Geometry check sheet. Reference: the model listing, model coordinates, mm. A direction names the side the tool comes from. Give positions to 0.01 mm unless a question says otherwise; leave off trailing zeros. Order: outer loops, then holes, each group sorted by start corner. A loop starts at its lowest first (then second) coordinate and runs counter-clockwise, first axis right, second up. Notation, with made-up numbers: M 84.25,88 L 99.25,88 A22 ccw 99.25,99 Z; hole C -25,66.25 d8. An arc over 180 degrees is marked long. One line per question, with ' | ' between items. Start each with the question number.
from build123d import *

# Parameters (mm, degrees)
SKETCH052_W     = 14
SKETCH052_H     = 6
PAD022_DEPTH    = 2
PAD023_DEPTH    = 1.8
PAD024_DEPTH    = 2
SKETCH056_W     = 3
SKETCH056_H     = 3
POCKET025_DEPTH = 2


with BuildPart() as part:
    # Sketch052 → Pad022 (new body)
    with BuildSketch(Plane(origin=(232, -0.5, 0.8), x_dir=(0, 1, 0), z_dir=(1, 0, 0))):
        with Locations((-52.22, 6.7)):
            Rectangle(SKETCH052_W, SKETCH052_H)
    extrude(amount=PAD022_DEPTH)

    # Sketch053 (on Face6 of Pad022) → Pad023 (join)
    with BuildSketch(Plane.YZ.offset(234)):
        with BuildLine():
            ThreePointArc((-54.97, 9.25), (-56.72, 7.5), (-54.97, 5.75))
            Line((-54.97, 5.75), (-50.47, 5.75))
            ThreePointArc((-50.47, 5.75), (-48.72, 7.5), (-50.47, 9.25))
            Line((-54.97, 9.25), (-50.47, 9.25))
        make_face()
    extrude(amount=PAD023_DEPTH)

    # Sketch054 (on Face11 of Pad023) → Pad024 (join)
    with BuildSketch(Plane.YZ.offset(235.8)):
        with BuildLine():
            ThreePointArc((-54.97, 8.5), (-55.97, 7.5), (-54.97, 6.5))
            Line((-54.97, 6.5), (-51.97, 6.5))
            ThreePointArc((-51.97, 6.5), (-50.97, 7.5), (-51.97, 8.5))
            Line((-54.97, 8.5), (-51.97, 8.5))
        make_face()
    extrude(amount=PAD024_DEPTH)

    # Sketch056 (on Face16 of Pad024) → Pocket025 (cut)
    with BuildSketch(Plane.YZ.offset(232)):
        with Locations((-53.47, 7.5)):
            Rectangle(SKETCH056_W, SKETCH056_H)
    extrude(amount=POCKET025_DEPTH, mode=Mode.SUBTRACT)


solid = part.part
Item 1: Depth check by flat-ended pin: pin 1 (2 mm diameter, centred on x = 237, z = 8.5, fed in from -Y); pin 2 (1 mm diameter, centred on x = 235, z = 7, fed in from +Y); pin 3 (0.6 mm diameter, centred on x = 237, y = -53, fed in from -Z). Enter the tip coordinate at first touch or a pass-through.
Item 2: Mould release check, pull along Z, two halves, no side actions. Record for faces 4 (the flat face through (233, -51.97, 7)), 5 (the flat face through (237.8, -54, 8)), 6 (the flat face through (233, -53, 9)), 7 (the cylindrical face through (234.89, -48.72, 7.46)): released by +Z, released by -Z, zero draft, split by the parting line, or undercut.
Item 3: Set-up check for faces 1 (the flat face through (237, -53, 6.5)), 2 (the cylindrical face through (234.89, -56.72, 7.54)), 3 (the flat face through (237, -53, 8.5)): record each of +Z, -Z, +X, -X, +Y, -Y from which the full face is reachable in a straight line by a thin tool's end or side.
Item 4: Cross-section at C-C, the plane z = 7.5. Record the cut outline in (x, y).
Item 5: Material ranges on line 1 along Y through (x, z) = (233.2, 7.05); line 2 along X through (y, z) = (-47, 5); line 3 along X through (y, z) = (-52.25, 6.2), recorded low to high.
Item 6: Cross-section at A-A, the plane x = 233.1. Record the cut outline in (y, z), plus the area to 3 significant figures.
Item 7: Cross-section at D-D, the plane x = 237.1. Record the cut outline in (y, z), plus the area to 3 significant figures.
Item 8: Cross-section at B-B, the plane y = -54.25. Record the cut outline in (x, z), plus the area to 3 significant figures.
Outcome:
1) pin 1: stops at y = -55.97 | pin 2: stops at y = -48.72 | pin 3: stops at z = 6.5
2) face 4: undercut | face 5: zero draft | face 6: undercut | face 7: split by the parting line
3) face 1: -Z, +X, +Y, -Y | face 2: +X, -Y | face 3: +Z, +X, +Y, -Y
4) outline: M 232,-59.72 L 234,-59.72 L 234,-56.72 L 235.8,-56.72 L 235.8,-55.97 L 237.8,-55.97 L 237.8,-50.97 L 235.8,-50.97 L 235.8,-48.72 L 234,-48.72 L 234,-45.72 L 232,-45.72 L 232,-51.97 L 234,-51.97 L 234,-54.97 L 232,-54.97 Z
5) line 1: y = -59.72 to -54.97, -51.97 to -45.72 | line 2: x = 232 to 234 | line 3: x = 234 to 235.8
6) outline: M -59.72,4.5 L -45.72,4.5 L -45.72,10.5 L -59.72,10.5 Z; hole M -54.97,6 L -51.97,6 L -51.97,9 L -54.97,9 Z | area: 75.0 mm²
7) outline: M -54.97,6.5 L -51.97,6.5 A1 ccw -51.97,8.5 L -54.97,8.5 A1 ccw Z | area: 9.14 mm²
8) outline: M 232,4.5 L 234,4.5 L 234,5.75 L 235.8,5.75 L 235.8,6.5 L 237.8,6.5 L 237.8,8.5 L 235.8,8.5 L 235.8,9.25 L 234,9.25 L 234,10.5 L 232,10.5 L 232,9 L 234,9 L 234,6 L 232,6 Z | area: 16.3 mm²
